```python
from build123d import *

# Parameters (mm, degrees)
F0_R     = 9.525
F1_DEPTH = 76.2
F2_R     = 1.651
F3_DEPTH = 12.7


with BuildPart() as f1:
    # F0 (on Front) → F1 (new body)
    with BuildSketch(Plane.XZ):
        with BuildLine():
            Line((-16.7763393044, 27.4915862828), (-16.7763393044, 9.313e-07))
            Line((-16.7763393044, 9.313e-07), (8.6236606956, 9.313e-07))
            Line((8.6236606956, 9.313e-07), (8.6236606956, 27.4915862828))
            ThreePointArc((8.6236606956, 27.4915862828), (-4.0763393044, 40.1915862828), (-16.7763393044, 27.4915862828))
        make_face()
        with Locations((-4.0763393044, 27.4915862828)):
            Circle(F0_R, mode=Mode.SUBTRACT)
        with Locations((-4.0763393044, 27.4915862828)):
            Circle(F0_R)
    extrude(amount=F1_DEPTH)

    # F2 (on face) → F3 (cut)
    with BuildSketch(Plane(origin=(0, 0, 9.313e-07), x_dir=(1, 0, 0), z_dir=(0, 0, -1))):
        with Locations((-10.4263393044, 6.35)):
            Circle(F2_R)
        with Locations((-10.4263393044, 69.85)):
            Circle(F2_R)
        with Locations((2.2736606956, 6.35)):
            Circle(F2_R)
        with Locations((2.2736606956, 69.85)):
            Circle(F2_R)
    extrude(amount=-F3_DEPTH, mode=Mode.SUBTRACT)


solid = f1.part
```
Can you work these out from the model? Positions are in its coordinate system, mm. A direction names the side the tool comes from. Give positions to 0.01 mm unless a question says otherwise; leave off trailing zeros. Loops run counter-clockwise (first coordinate to the right, second up) from the corner with the lowest first, then second, coordinate; pieces in that order, holes last. Notation, with made-up numbers: M 13.5,-18.5 L 34.5,-18.5 A16 ccw 34.5,6.5 Z; hole C -2,82.5 d1. An arc over 180 degrees is marked long. Use CSV: the item, a comma, the result in double quotes. Start each with the question number.
1. On a 3-axis mill with a long thin cutter (end or side, diameter ignored), from which of +Z, -Z, +X, -X, +Y, -Y can I reach the whole of each face in a straight line? I mean faces 1 (the face through (-10, -70, 12.7)), 2 (the face through (-4, -38, 0)). Say none if no direction works.
2. If we mould it in two halves opening along X, with no side actions, what happens to faces 3 (the face through (-9.539, -7.742, 6.261)), 4 (the face through (-4, 0, 20)), 5 (the face through (8.624, -38, 14)), 6 (the face through (-3.8, -37.57, 40.19))? For each: released by +X, released by -X, zero draft, split by the parting line, or undercut.
3. Imagine slicing it at C-C, the plane x = -14.75. Write out the boundary of the cut face in (y, z), plus the area to 3 significant figures.
4. Imagine slicing it at B-B, the plane y = -69.85. Write out the boundary of the cut face in (x, z), plus the area to 3 significant figures.
5. For P1, Ø2.5, axis at x = 2.27, y = -69.85, coming from the -Z side; P2, Ø3, axis at x = 2.27, y = -6.35, coming from the +Z side; P3, Ø2, axis at x = -10.43, y = -69.85, coming from the +Z side, each with a flat end and sliding along its axis, tell me the tip position at first contact or that it passes through.
6. Imagine slicing it at D-D, the plane y = -35. Write out the boundary of the cut face in (x, z), plus the area to 3 significant figures.
7. If I drill on L1, parallel to X at y = -69.85, z = 3.75; L2, parallel to Y at x = -11.5, z = 10.5; L3, parallel to Y at x = 3.5, z = 3, over which ranges is the centre line in solid material (lowest first)?
8. Imagine slicing it at A-A, the plane z = 4. Write out the boundary of the cut face in (x, y).
Response values:
1,face 1,"-Z"
1,face 2,"-Z, +X, -X, +Y, -Y"
2,face 3,"undercut"
2,face 4,"zero draft"
2,face 5,"released by +X"
2,face 6,"split by the parting line"
3,outline,"M -76.2,0 L 0,0 L 0,34.37 L -76.2,34.37 Z"
3,area,"2,620 mm^2"
4,outline,"M -16.78,0 L -12.08,0 L -12.08,12.7 L -8.78,12.7 L -8.78,0 L 0.62,0 L 0.62,12.7 L 3.92,12.7 L 3.92,0 L 8.62,0 L 8.62,27.49 A12.7 ccw -16.78,27.49 Z"
4,area,"868 mm^2"
5,P1,"z = 12.7"
5,P2,"z = 39.23"
5,P3,"z = 39.01"
6,outline,"M -16.78,0 L 8.62,0 L 8.62,27.49 A12.7 ccw -16.78,27.49 Z"
6,area,"952 mm^2"
7,L1,"-16.78 to -12.08, -8.78 to 0.62, 3.92 to 8.62"
7,L2,"-76.2 to -71.1, -68.6 to -7.6, -5.1 to 0"
7,L3,"-76.2 to -70.96, -68.74 to -7.46, -5.24 to 0"
8,outline,"M -16.78,-76.2 L 8.62,-76.2 L 8.62,0 L -16.78,0 Z; hole C -10.43,-69.85 d3.3; hole C -10.43,-6.35 d3.3; hole C 2.27,-69.85 d3.3; hole C 2.27,-6.35 d3.3"
